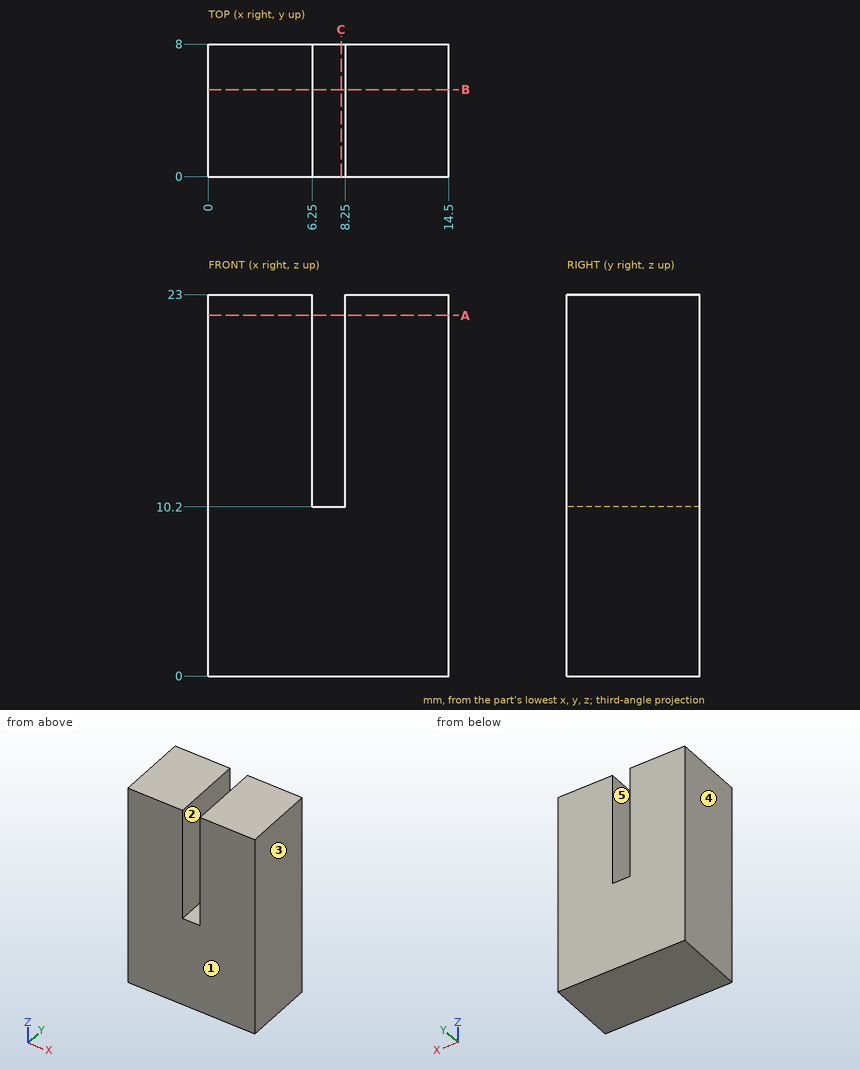
Geometry: see drawing. Coordinates: mm, zero at the bounding-box minimum. A direction names the side the tool comes from. Give positions to 0.01 mm unless a question says otherwise; leave off trailing zeros. Order: outer loops, then holes, each group sorted by start corner. A loop starts at its lowest first (then second) coordinate and runs counter-clockwise, first axis right, second up. Notation, with made-up numbers: (28.5, 66.5) -> (85.5, 66.5) arc R24 ccw to (85.5, 88.5) -> close; hole circle Ø6 at (52, -28.5). An arc over 180 degrees is marked (long way). Write item = value, one per line.
Q1. Material intervals for line 1 (X direction, y = 3.5, z = 17.75); line 2 (Z direction, x = 7.5, y = 0.5), sorted ascending. Write a range as from..to.
Data:
line_1 = 0..6.25, 8.25..14.5
line_2 = 0..10.2
Q2. Cut plane A-A, the plane z = 21.75. Output: boundary loops of the cut face in (x, y).
Data:
outline = (0, 0) -> (6.25, 0) -> (6.25, 8) -> (0, 8) -> close; (8.25, 0) -> (14.5, 0) -> (14.5, 8) -> (8.25, 8) -> close
Q3. Pull-direction query (X, two-part tool) for the marked faces 1, 2 and 3; classes: released by +X, released by -X, zero draft, split by the parting line, or undercut.
Data:
face_1 = zero draft
face_2 = undercut
face_3 = released by +X
Q4. Cut plane B-B, the plane y = 5.25. Output: boundary loops of the cut face in (x, z).
Data:
outline = (0, 0) -> (14.5, 0) -> (14.5, 23) -> (8.25, 23) -> (8.25, 10.2) -> (6.25, 10.2) -> (6.25, 23) -> (0, 23) -> close
Q5. Set-up query: the marked faces 4 and 5. Return all of +Z, -Z, +X, -X, +Y, -Y with unobstructed straight access to the full face (end or side cutting, diameter ignored); none if empty.
Data:
face_4 = +Z, -Z, -X, +Y, -Y
face_5 = +Z, +Y, -Y
Q6. Cut plane C-C, the plane x = 8. Output: boundary loops of the cut face in (y, z), and give its area (3 significant figures).
Data:
outline = (0, 0) -> (8, 0) -> (8, 10.2) -> (0, 10.2) -> close
area = 81.6 mm^2
Q7. Pin query (flat end, axial travel): pin 1 (0.6 mm diameter, centred on x = 7, y = 2, fed in from +Z). Return the tip coordinate at first contact, or that it passes through.
Data:
pin_1 = 10.2
